Build history of the part. All positions in model axes, mm. A direction names the side the tool comes from. Coordinates: 2 decimals unless noted, no trailing zeros. Loops run counter-clockwise (first coordinate to the right, second up) from the corner with the lowest first, then second, coordinate; pieces in that order, holes last.
(1) Slice it at D-D (x = -5.5). Give the cut face in (y, z), and give its area (3 significant figures).
(2) Two-plate mould, pull along X, no slides. Class faces 1 (the face through (5.446, 0.811, -14.809)), 2 (the face through (1, 1, 0)), 3 (the face through (0.715, 0.811, -10.301)): pulls with the +X half, pulls with the -X half, needs draft (parallel to the pull), parting line crosses it, or undercut.
(3) Tool access for faces 4 (the face through (5, 1, -16)), 5 (the face through (4.99, 0.811, -12.375)), 6 (the face through (1, 1, -13)): list every direction of +Z, -Z, +X, -X, +Y, -Y with a clear straight run to the whole face (end or side of a thin tool).
(4) Wall check: L1, parallel to X at y = 0.6, z = -14.75; L2, parallel to X at y = 0.95, z = -5; L3, parallel to Z at x = -7, y = 1.15. Give the ranges that are in metal, low to high.
(5) Slice it at C-C (y = 0.2). Give the cut face in (x, z) (3 decimals).
(6) Slice it at B-B (z = -5). Give the cut face in (x, y), and give its area (3 significant figures).
(7) Slice it at A-A (x = 6). Give the cut face in (y, z).
from build123d import *

# Parameters (mm, degrees)
SKETCH1_R           = 2.05
BOSS_EXTRUDE1_DEPTH = 1.6
SKETCH2_R           = 0.45
CUT_EXTRUDE1_DEPTH  = 19.935680606
FILLET1_R           = 1


with BuildPart() as part:
    # Sketch1 → Boss-Extrude1 (new body)
    with BuildSketch(Plane(origin=(0, 0, 0), x_dir=(1, 0, 0), z_dir=(0, 1, 0))):
        Polygon((1, 10), (1, 16), (10, 16), (10, 8), (10, 0), (0, 0), (-8, 0), (-8, 10), align=None)
        with Locations(Location((6, 5, 0), (0, 0, 270))):
            Circle(SKETCH1_R, mode=Mode.SUBTRACT)
    extrude(amount=BOSS_EXTRUDE1_DEPTH)

    # Sketch2 → Cut-Extrude1 (cut, through all)
    with BuildSketch(Plane(origin=(0, 1.6, 0), x_dir=(1, 0, 0), z_dir=(0, 1, 0))):
        with Locations(Location((5, 14.75, 0), (0, 0, 270))):
            Circle(SKETCH2_R)
        with BuildLine():
            Line((4.55, 11.575), (4.55, 11.925))
            ThreePointArc((4.55, 11.925), (5, 12.375), (5.45, 11.925))
            Line((5.45, 11.925), (5.45, 11.575))
            ThreePointArc((5.45, 11.575), (5, 11.125), (4.55, 11.575))
        make_face()
    extrude(amount=-CUT_EXTRUDE1_DEPTH, mode=Mode.SUBTRACT)

    # Fillet1
    fillet1_edges = [part.edges().sort_by_distance(p)[0] for p in [
        (1, 0.8, -10),
    ]]
    fillet(fillet1_edges, radius=FILLET1_R)


solid = part.part
Response values:
1. outline: (0, -10) - (1.6, -10) - (1.6, 0) - (0, 0) - close
1. area: 16.0 mm2
2. face 1: undercut
2. face 2: needs draft
2. face 3: pulls with the -X half
3. face 4: -Z, +X, -X, +Y, -Y
3. face 5: +Y, -Y
3. face 6: -Z, -X, +Y, -Y
4. L1: x = 1 to 4.55, 5.45 to 10
4. L2: x = -8 to 3.95, 8.05 to 10
4. L3: z = -10 to 0
5. outline: (-8, -10) - (0, -10) arc R1 cw to (1, -11) - (1, -16) - (10, -16) - (10, 0) - (-8, 0) - close; hole circle Ø4.1 at (6, -5); hole circle Ø0.9 at (5, -14.75); hole (4.55, -11.925) arc R0.45 ccw to (5.45, -11.925) - (5.45, -11.575) arc R0.45 ccw to (4.55, -11.575) - close
6. outline: (-8, 0) - (3.95, 0) - (3.95, 1.6) - (-8, 1.6) - close; (8.05, 0) - (10, 0) - (10, 1.6) - (8.05, 1.6) - close
6. area: 22.2 mm2
7. outline: (0, -16) - (1.6, -16) - (1.6, -7.05) - (0, -7.05) - close; (0, -2.95) - (1.6, -2.95) - (1.6, 0) - (0, 0) - close
